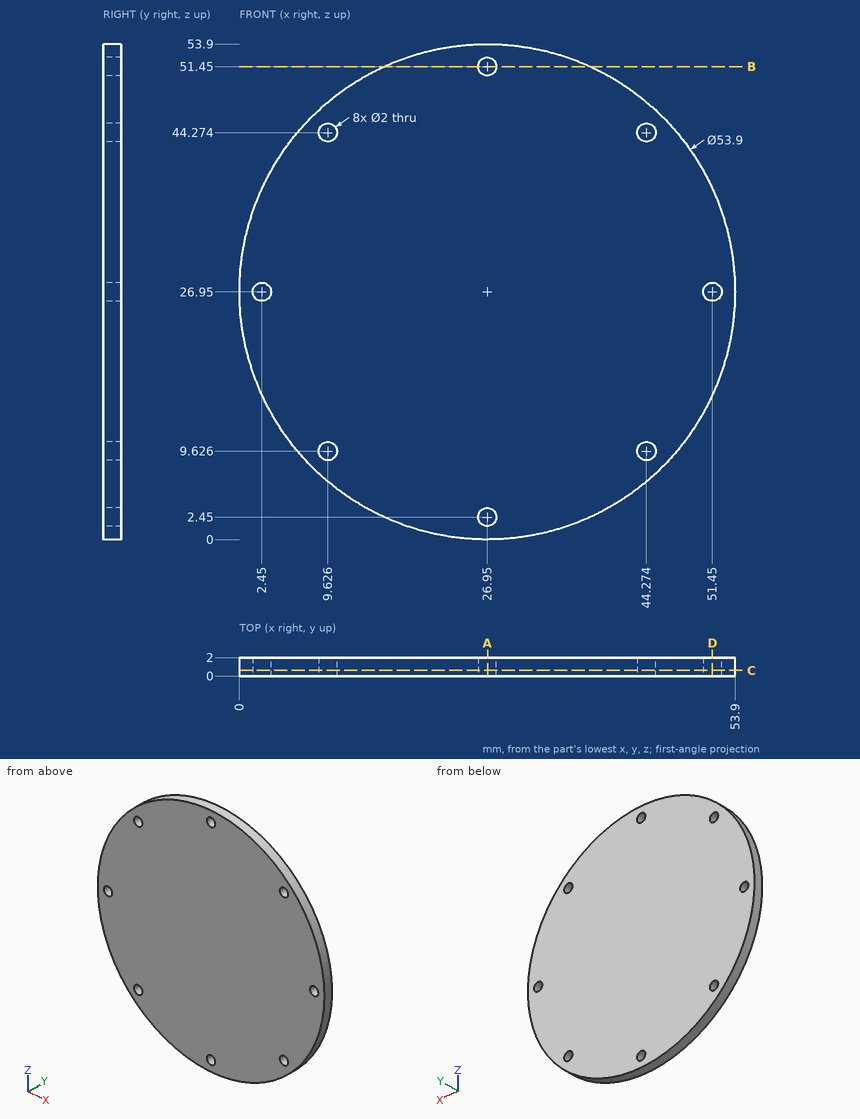
Design review of the part shown in the three views and the two pictorial views. Dimensions are in mm from the part's minimum x, y and z. Give positions to 0.01 mm unless a question says otherwise; leave off trailing zeros. Write each loop counter-clockwise with the first axis right and the second up, starting at its lowest first coordinate (ties: lowest second). Pieces come first, ordered by that corner, then holes. Notation, with made-up numbers: (-28.75, 13.5) - (26.25, 13.5) arc R24 ccw to (26.25, 45.5) - close; hole circle Ø7 at (72.25, -26.75). An arc over 180 degrees is marked (long way). Return JSON: item names as keys, results as strings. Group by question number.
(1) We need section B-B, the plane z = 51.45. Give the boundary of the cut face in (x, y), then the cut area to 3 significant figures.
(2) We need section D-D, the plane x = 51.45. Give the boundary of the cut face in (y, z).
(3) We need section C-C, the plane y = 0.6. Give the number of separate pieces and of enclosed holes in the cut face, then the cut area to 3 significant figures.
(4) To check wall thickness, follow probe 1 along X at (y, z) = (1.7, 27); probe 2 along X at (y, z) = (0.65, 9). State the ranges of each line that lie inside material, in increasing order.
(5) We need section A-A, the plane x = 27. Give the boundary of the cut face in (y, z), then the cut area to 3 significant figures.
(6) Insertion check: pin 1 (1 mm diameter, centred on x = 30.5, y = 0.5, fed in from -Z). The pin has a flat end and moves straight along its axis. Give the tip position at first contact, or say it passes through.
Reported:
{
 "1": {"outline": "(15.72, 0) - (25.95, 0) - (25.95, 2) - (15.72, 2) - close; (27.95, 0) - (38.18, 0) - (38.18, 2) - (27.95, 2) - close", "area": "40.9 mm2"},
 "2": {"outline": "(0, 15.72) - (2, 15.72) - (2, 25.95) - (0, 25.95) - close; (0, 27.95) - (2, 27.95) - (2, 38.18) - (0, 38.18) - close"},
 "3": {"separate pieces": "1", "enclosed holes": "8", "area": "2,260 mm2"},
 "4": {"probe 1": "x = 0 to 1.45, 3.45 to 50.45, 52.45 to 53.9", "probe 2": "x = 6.85 to 8.85, 10.41 to 43.49, 45.05 to 47.05"},
 "5": {"outline": "(0, 0) - (2, 0) - (2, 1.45) - (0, 1.45) - close; (0, 3.45) - (2, 3.45) - (2, 50.45) - (0, 50.45) - close; (0, 52.45) - (2, 52.45) - (2, 53.9) - (0, 53.9) - close", "area": "99.8 mm2"},
 "6": {"pin 1": "stops at z = 0.17"}
}
